Geometry: final body of the model. Coordinates: model frame, mm. Coordinates: 2 decimals unless noted, no trailing zeros. Order: outer loops, then holes, each group sorted by start corner. A loop starts at its lowest first (then second) coordinate and runs counter-clockwise, first axis right, second up. Notation, with made-up numbers: (54.5, -25.75) -> (87.5, -25.75) arc R25 cw to (87.5, 13.25) -> close; hole circle Ø5 at (-13.5, 43). An arc over 180 degrees is marked (long way). Answer in a Markdown table with one row per item. Add a question column.
1) Pull-direction query (Y, two-part tool) for faces 1 (the face through (-72.075, -69.314, 0.986)), 2 (the face through (-1, 1, 2)); classes: +Y half, -Y half, draft (parallel to the pull), parting line (faces both ways), or undercut.
2) Section query B-B on z = 0.65. Return the cut outline in (x, y).
3) Section query A-A on x = 12.5. Return the cut outline in (y, z).
4) Section query C-C on y = -71. Return the cut outline in (x, z), then the cut area to 3 significant figures.
5) Ray query, line 1 (Y direction, x = 71, z = 1.35); line 2 (Y direction, x = -19.5, z = 1). Return the intervals inside material, ascending. Write a range as from..to.
Autodesk Fusion 360 part; units mm, degrees
sketch "Sketch1" plane through (0, 0, 0) normal (0, 0, 1) x (1, 0, 0)
  line L0 (75, 75) -> (-75, 75)
  line L1 (-75, 75) -> (-75, -75)
  line L2 (-75, -75) -> (75, -75)
  line L3 (75, -75) -> (75, 75)
  line L4 (75, 75) -> (-75, -75) construction
  line L5 (-75, 75) -> (75, -75) construction
  dimension "d1" = 150
  dimension "d2" = 150
extrude "Extrude1" add sketch "Sketch1" along normal blind 1
sketch "Sketch2" plane through (0, 0, 1) normal (0, 0, 1) x (-1, 0, 0)
  line L0 (-75, 75) -> (-75, -75)
  line L1 (-75, -75) -> (75, -75)
  line L2 (75, -75) -> (75, 75)
  line L3 (75, 75) -> (-75, 75)
  line L4 (-75, -75) -> (-71, -75)
  line L5 (-71, -75) -> (-71, -71)
  line L6 (-71, -71) -> (-75, -71)
  line L7 (-75, -71) -> (-75, -75)
  circle A0 centre (-71, -71) radius 2
  dimension "d5" = 4
  dimension "d6" = 4
  dimension "d7" = 4
extrude "Extrude2" cut sketch "Sketch2" against normal blind 1 contours L5 L6 A0 | L5 L6 A0
sketch "Sketch3" plane through (0, 0, 1) normal (0, 0, 1) x (-1, 0, 0)
  circle A0 centre (-71, -71) radius 2
  line L0 (-75, 75) -> (-75, -75)
  line L1 (-75, -75) -> (75, -75)
  line L2 (75, -75) -> (75, 75)
  line L3 (75, 75) -> (-75, 75)
  line L4 (75, -75) -> (71, -75)
  line L5 (71, -75) -> (71, -71)
  line L6 (71, -71) -> (75, -71)
  line L7 (75, -71) -> (75, -75)
  line L8 (75, 75) -> (71, 75)
  line L9 (71, 75) -> (71, 71)
  line L10 (71, 71) -> (75, 71)
  line L11 (75, 71) -> (75, 75)
  line L12 (-75, 75) -> (-71, 75)
  line L13 (-71, 75) -> (-71, 71)
  line L14 (-71, 71) -> (-75, 71)
  line L15 (-75, 71) -> (-75, 75)
  circle A1 centre (-71, 71) radius 2
  circle A2 centre (71, 71) radius 2
  circle A3 centre (71, -71) radius 2
  dimension "d10" = 4
  dimension "d11" = 4
  dimension "d12" = 4
  dimension "d13" = 4
  dimension "d14" = 4
  dimension "d15" = 4
  dimension "d16" = 4
  dimension "d17" = 4
  dimension "d18" = 4
extrude "Extrude3" cut sketch "Sketch3" against normal blind 1 contours L13 L14 A1 | L13 L14 A1 | L9 L10 A2 | L9 L10 A2 | L5 L6 A3 | L5 L6 A3
sketch "Sketch4" plane through (0, 0, 1) normal (0, 0, 1) x (-1, 0, 0)
  circle A0 centre (71, -71) radius 2
  circle A1 centre (71, 71) radius 2
  circle A2 centre (-71, 71) radius 2
  circle A3 centre (-71, -71) radius 2
  line L0 (-75, 75) -> (-75, -75)
  line L1 (-75, -75) -> (75, -75)
  line L2 (75, -75) -> (75, 75)
  line L3 (75, 75) -> (-75, 75)
  line L4 (0, 75) -> (0, 60)
  line L5 (0, 60) -> (-36, 60)
  line L6 (-36, 60) -> (36, 60)
  line L7 (36, 60) -> (36, 35)
  line L8 (36, 35) -> (-36, 35)
  line L9 (-36, 35) -> (-36, 60)
  dimension "d21" = 15
  dimension "d24" = 72
extrude "Extrude4" cut sketch "Sketch4" against normal blind 1 contours L5 L6 L7 L8 L9
extrude "Extrude5" add 1 faces at (-12, 35.1244, 1) along direction (0, 0, 1) blind 1
Result:
| question | item | result |
|---|---|---|
| 1 | face 1 | undercut |
| 1 | face 2 | draft |
| 2 | outline | (-75, -75) -> (75, -75) -> (75, 75) -> (-75, 75) -> close; hole circle Ø4 at (-71, -71); hole circle Ø4 at (-71, 71); hole (-36, -60) -> (36, -60) -> (36, -35) -> (-36, -35) -> close; hole circle Ø4 at (71, -71); hole circle Ø4 at (71, 71) |
| 3 | outline | (-75, 0) -> (-60, 0) -> (-60, 2) -> (-75, 2) -> close; (-35, 0) -> (75, 0) -> (75, 2) -> (-35, 2) -> close |
| 4 | outline | (-75, 0) -> (-73, 0) -> (-73, 2) -> (-75, 2) -> close; (-69, 0) -> (69, 0) -> (69, 2) -> (-69, 2) -> close; (73, 0) -> (75, 0) -> (75, 2) -> (73, 2) -> close |
| 4 | area | 284 mm2 |
| 5 | line 1 | -75..-73, -69..69, 73..75 |
| 5 | line 2 | -75..-60, -35..75 |
